Geometry check sheet. Reference: the model listing, model coordinates, mm. A direction names the side the tool comes from. Round coordinates to 2 decimals unless told otherwise and drop trailing zeros. Order: outer loops, then holes, each group sorted by start corner. A loop starts at its lowest first (then second) coordinate and runs counter-clockwise, first axis right, second up. Notation, with made-up numbers: (17.5, 14) - (39.5, 14) arc R5 cw to (39.5, 21) - close; hole circle Ø1 at (7.25, -7.5). An arc over 180 degrees is marked (long way). Write each question's results on one line, items separated by ' | '.
```python
from build123d import *

# Parameters (mm, degrees)
BOSS_EXTRUDE1_DEPTH   = 10.7
SKETCH1_4_R           = 1
BOSS_EXTRUDE5_DEPTH   = 9.5
BOSS_EXTRUDE5_2_DEPTH = 9.5
BOSS_EXTRUDE3_DEPTH   = 2.5
DOME1_FACE_RADIUS     = 1
DOME1_HEIGHT          = 0.95
DOME2_FACE_RADIUS     = 1
DOME2_HEIGHT          = 0.95
CUT_EXTRUDE1_DEPTH    = 13.121494339
SKETCH5_R             = 1.2
BOSS_EXTRUDE6_DEPTH   = 6.5
SKETCH6_R             = 0.65
CUT_EXTRUDE2_DEPTH    = 4
CUT_EXTRUDE3_START    = -2.34
CUT_EXTRUDE3_DEPTH    = 2.34


with BuildPart() as part:
    # Sketch1 → Boss-Extrude1 (new body)
    with BuildSketch(Plane.XY):
        with BuildLine():
            Line((0, -2.625), (0, 2.625))
            Line((0, 2.625), (8.575, 2.625))
            ThreePointArc((8.575, 2.625), (9.724048519, 2.149048519), (10.2, 1))
            Line((10.2, 1), (10.2, -1))
            ThreePointArc((10.2, -1), (9.724048519, -2.149048519), (8.575, -2.625))
            Line((8.575, -2.625), (0, -2.625))
        make_face()
        Polygon((0.5, -2.125), (8.367893219, -2.125), (9.7, -0.792893219), (9.7, 0.792893219), (8.367893219, 2.125), (0.5, 2.125), align=None, mode=Mode.SUBTRACT)
    extrude(amount=BOSS_EXTRUDE1_DEPTH)

    # Sketch3 → Boss-Extrude3 (add)
    with BuildSketch(Plane(origin=(0, 0, 1), x_dir=(-1, 0, 0), z_dir=(0, 0, -1))):
        Polygon((-0.5, -2.125), (-0.5, 2.125), (-8.367893219, 2.125), (-9.7, 0.792893219), (-9.7, -0.792893219), (-8.367893219, -2.125), align=None)
    extrude(amount=-BOSS_EXTRUDE3_DEPTH)



with BuildPart() as body_2:
    # Sketch1<4> → Boss-Extrude5 (new body)
    with BuildSketch(Plane.XY):
        with Locations((2.6, 0)):
            Circle(SKETCH1_4_R)
    extrude(amount=BOSS_EXTRUDE5_DEPTH)

    # Dome2: a dome of height H over a round flat face of radius A is a cap of a sphere of radius (A * A + H * H) / (2 * H)
    dome2_r = (DOME2_FACE_RADIUS * DOME2_FACE_RADIUS + DOME2_HEIGHT * DOME2_HEIGHT) / (2 * DOME2_HEIGHT)
    dome2_base = Plane((2.6, 0, 9.5), z_dir=(0, 0, 1))
    with Locations(dome2_base.offset(DOME2_HEIGHT - dome2_r)):
        dome2_ball = Sphere(dome2_r, mode=Mode.PRIVATE)
    add(split(dome2_ball, bisect_by=dome2_base, keep=Keep.TOP, mode=Mode.PRIVATE))


with BuildPart() as body_3:
    # Sketch1<4> → Boss-Extrude5 2 (new body)
    with BuildSketch(Plane.XY):
        with Locations(Location((7.6, 0, 0), (0, 0, 180))):
            Circle(SKETCH1_4_R)
    extrude(amount=BOSS_EXTRUDE5_2_DEPTH)

    # Dome1: a dome of height H over a round flat face of radius A is a cap of a sphere of radius (A * A + H * H) / (2 * H)
    dome1_r = (DOME1_FACE_RADIUS * DOME1_FACE_RADIUS + DOME1_HEIGHT * DOME1_HEIGHT) / (2 * DOME1_HEIGHT)
    dome1_base = Plane((7.6, 0, 9.5), z_dir=(0, 0, 1))
    with Locations(dome1_base.offset(DOME1_HEIGHT - dome1_r)):
        dome1_ball = Sphere(dome1_r, mode=Mode.PRIVATE)
    add(split(dome1_ball, bisect_by=dome1_base, keep=Keep.TOP, mode=Mode.PRIVATE))


with BuildPart() as cut_extrude1_tool:
    # Sketch4 → Cut-Extrude1 (new, through all)
    with BuildSketch(Plane.XY.offset(6)):
        with BuildLine():
            Line((7.475, 0.992156742), (7.475, 0.125))
            Line((7.475, 0.125), (6.607843258, 0.125))
            ThreePointArc((6.607843258, 0.125), (6.6, 0), (6.607843258, -0.125))
            Line((6.607843258, -0.125), (7.475, -0.125))
            Line((7.475, -0.125), (7.475, -0.992156742))
            ThreePointArc((7.475, -0.992156742), (7.6, -1), (7.725, -0.992156742))
            Line((7.725, -0.992156742), (7.725, -0.125))
            Line((7.725, -0.125), (8.592156742, -0.125))
            ThreePointArc((8.592156742, -0.125), (8.6, 0), (8.592156742, 0.125))
            Line((8.592156742, 0.125), (7.725, 0.125))
            Line((7.725, 0.125), (7.725, 0.992156742))
            ThreePointArc((7.725, 0.992156742), (7.6, 1), (7.475, 0.992156742))
        make_face()
        with BuildLine():
            Line((3.592156742, -0.125), (2.725, -0.125))
            Line((2.725, -0.125), (2.725, -0.992156742))
            ThreePointArc((2.725, -0.992156742), (2.6, -1), (2.475, -0.992156742))
            Line((2.475, -0.992156742), (2.475, -0.125))
            Line((2.475, -0.125), (1.607843258, -0.125))
            ThreePointArc((1.607843258, -0.125), (1.6, 0), (1.607843258, 0.125))
            Line((1.607843258, 0.125), (2.475, 0.125))
            Line((2.475, 0.125), (2.475, 0.992156742))
            ThreePointArc((2.475, 0.992156742), (2.6, 1), (2.725, 0.992156742))
            Line((2.725, 0.992156742), (2.725, 0.125))
            Line((2.725, 0.125), (3.592156742, 0.125))
            ThreePointArc((3.592156742, 0.125), (3.6, 0), (3.592156742, -0.125))
        make_face()
    extrude(amount=CUT_EXTRUDE1_DEPTH)


with BuildPart() as body_2_1:
    add(body_2.part)

    # Cut-Extrude1: cut by cut_extrude1_tool
    add(cut_extrude1_tool.part, mode=Mode.SUBTRACT)


with BuildPart() as body_3_1:
    add(body_3.part)

    # Cut-Extrude1: cut by cut_extrude1_tool
    add(cut_extrude1_tool.part, mode=Mode.SUBTRACT)


with BuildPart() as part_1:
    add(part.part)

    add(body_2_1.part)  # Boss-Extrude6 merges body 2

    add(body_3_1.part)  # Boss-Extrude6 merges body 3
    # Sketch5 → Boss-Extrude6 (add)
    with BuildSketch(Plane.XY.offset(3.5)):
        with Locations((7.6, 0)):
            Circle(SKETCH5_R)
        with Locations((2.6, 0)):
            Circle(SKETCH5_R)
    extrude(amount=-BOSS_EXTRUDE6_DEPTH)

    # Sketch6 → Cut-Extrude2 (cut)
    with BuildSketch(Plane(origin=(0, 0, -3), x_dir=(-1, 0, 0), z_dir=(0, 0, -1))):
        with Locations((-2.6, 0)):
            Circle(SKETCH6_R)
        with Locations((-7.6, 0)):
            Circle(SKETCH6_R)
    extrude(amount=-CUT_EXTRUDE2_DEPTH, mode=Mode.SUBTRACT)

    # Sketch7 → Cut-Extrude3 (cut)
    with BuildSketch(Plane(origin=(0, 0, -3), x_dir=(-1, 0, 0), z_dir=(0, 0, -1)).offset(CUT_EXTRUDE3_START)):
        with BuildLine():
            Line((-2.6, -0.65), (-2.6, -1.2))
            ThreePointArc((-2.6, -1.2), (-1.751471863, -0.848528137), (-1.4, 0))
            ThreePointArc((-1.4, 0), (-1.751471863, 0.848528137), (-2.6, 1.2))
            Line((-2.6, 1.2), (-2.6, 0.65))
            ThreePointArc((-2.6, 0.65), (-2.140380592, 0.459619408), (-1.95, 0))
            ThreePointArc((-1.95, 0), (-2.140380592, -0.459619408), (-2.6, -0.65))
        make_face()
        with BuildLine():
            ThreePointArc((-7.6, 1.2), (-8.8, 0), (-7.6, -1.2))
            Line((-7.6, -1.2), (-7.6, 1.2))
        make_face()
    extrude(amount=CUT_EXTRUDE3_DEPTH, mode=Mode.SUBTRACT)


solid = part_1.part
```
(1) Draft check along Y on faces 4 (the face through (10.2, 0, 5)), 5 (the face through (5, 0, 3.5)), 6 (the face through (4, 2.625, 5)). Enter one of: released by +Y, released by -Y, zero draft, split by the parting line, or undercut.
Answers follow:
face 4: zero draft | face 5: undercut | face 6: released by +Y
(2) Section check B-B (z = -2). Record the cut outline in (x, y).
Answers follow:
outline: (2.6, -1.2) arc R1.2 ccw to (2.6, 1.2) - (2.6, 0.65) arc R0.65 cw to (2.6, -0.65) - close; (7.6, -1.2) - (7.6, -0.65) arc R0.65 cw to (7.6, 0.65) - (7.6, 1.2) arc R1.2 ccw to start
(3) Access from +Z, -Z, +X, -X, +Y, -Y to the whole of each face (thin tool, end or side, straight path). Record for faces 1 (the face through (3.524, -0.383, 6.458)), 2 (the face through (9.737, -2.136, 5.275)), 3 (the face through (0.5, 0, 0.5)).
Answers follow:
face 1: +Z | face 2: +Z, -Z, +X, -Y | face 3: -Z
(4) Section check A-A (z = 5). Record the cut outline in (x, y) (3 decimals).
Answers follow:
outline: (0, -2.625) - (8.575, -2.625) arc R1.625 ccw to (10.2, -1) - (10.2, 1) arc R1.625 ccw to (8.575, 2.625) - (0, 2.625) - close; circle Ø2 at (2.6, 0); circle Ø2 at (7.6, 0); hole (0.5, -2.125) - (8.368, -2.125) - (9.7, -0.793) - (9.7, 0.793) - (8.368, 2.125) - (0.5, 2.125) - close
(5) Section check D-D (z = 8.5). Give the number of separate pieces and of enclosed holes in the cut face, then the cut area to 3 significant figures.
Answers follow:
separate pieces: 9 | enclosed holes: 1 | area: 19.5 mm²
(6) Depth check by flat-ended pin: pin 1 Ø2 at (x, y) = (2.6, 0) entering from -Z; pin 2 Ø2 at (x, y) = (8, 0) entering from +Z; pin 3 Ø0.6 at (y, z) = (-1, -1.5) entering from -X; pin 4 Ø0.6 at (y, z) = (-1, -2.5) entering from +X. Enter the tip coordinate at first touch or a pass-through.
Answers follow:
pin 1: z = -3 | pin 2: z = 10.43 | pin 3: x = 2.6 | pin 4: x = 7.6
(7) Material ranges on line 1 (Y direction, x = 2.5, z = 4.25) (3 decimals); line 2 (Y direction, x = 7.6, z = 0.05) (3 decimals); line 3 (Y direction, x = 8.5, z = 4.5) (3 decimals), recorded low to high.
Answers follow:
line 1: -2.625 to -2.125, -0.995 to 0.995, 2.125 to 2.625 | line 2: -2.625 to -2.125, -1.2 to -0.65, 0.65 to 1.2, 2.125 to 2.625 | line 3: -2.625 to -1.993, -0.436 to 0.436, 1.993 to 2.625
(8) Section check C-C (x = 6). Record the cut outline in (y, z) (3 decimals), then the cut area to 3 significant figures.
Answers follow:
outline: (-2.625, 0) - (-2.125, 0) - (-2.125, 1) - (2.125, 1) - (2.125, 0) - (2.625, 0) - (2.625, 10.7) - (2.125, 10.7) - (2.125, 3.5) - (-2.125, 3.5) - (-2.125, 10.7) - (-2.625, 10.7) - close | area: 21.3 mm²
